Could you check a few things on this model? Use its own coordinates, in mm. Give positions to 0.01 mm unless a question says otherwise; leave off trailing zeros. Loops run counter-clockwise (first coordinate to the right, second up) from the corner with the lowest first, then second, coordinate; pieces in that order, holes last. Notation, with made-up numbers: M 44.5,43.5 L 60.5,43.5 A23 cw 60.5,51.5 Z; hole C 76.25,65 d5. An arc over 180 degrees is marked long. Answer in a Markdown table with one row per item. Add a question column.
1. I'm going to push flat-ended pins straight in: pin 1 Ø1 at (y, z) = (1, -4) entering from -X; pin 2 Ø1.5 at (x, z) = (5.5, -2.5) entering from -Y; pin 3 Ø1 at (y, z) = (2.5, -6.5) entering from +X. Where does each tip first touch, or does it pass through?
2. If we section it at D-D on x = 16: List the corners of the cut face in (y, z) for me, then the cut area to 3 significant figures.
3. I need wall thicknesses on line 1 along X through (y, z) = (1.8, 0); line 2 along X through (y, z) = (1.9, 1.5); line 3 along Z through (x, y) = (-16.5, 1.75). Which ranges of each line are inside material? Lowest first, please. Write a range as from..to.
4. If we section it at B-B on z = 0: List the corners of the cut face in (x, y) for me, then the cut area to 4 significant figures.
5. Thinking about a two-plate mould opening in X: for faces 1 (the cylindrical face through (19.83, 1.52, -8.44)), 2 (the cylindrical face through (19, 2, 0)), 3 (the cylindrical face through (-19.83, 1.52, -8.44)), which applies, released by +X, released by -X, zero draft, split by the parting line, or undercut?
6. If we section it at A-A on y = 1.3: List the corners of the cut face in (x, z) for me, then the cut area to 3 significant figures.
7. If we section it at C-C on x = -18: List the corners of the cut face in (y, z) for me, then the cut area to 3 significant figures.
```python
from build123d import *

# Parameters (mm, degrees)
ESBO_O1_W                = 44.5
ESBO_O1_H                = 22
RESSALTO_EXTRUS_O1_DEPTH = 3
FILETE1_R                = 8.5
ESBO_O2_R                = 2
CORTE_EXTRUS_O1_DEPTH    = 26.001249969


with BuildPart() as part:
    # Esboço1 → Ressalto-extrusão1 (new body)
    with BuildSketch(Plane(origin=(0, 0, 0), x_dir=(1, 0, 0), z_dir=(0, 1, 0))):
        Rectangle(ESBO_O1_W, ESBO_O1_H)
    extrude(amount=RESSALTO_EXTRUS_O1_DEPTH)

    # Filete1
    filete1_edges = [part.edges().sort_by_distance(p)[0] for p in [
        (22.25, 1.5, 11),
        (-22.25, 1.5, 11),
        (-22.25, 1.5, -11),
        (22.25, 1.5, -11),
    ]]
    fillet(filete1_edges, radius=FILETE1_R)

    # Esboço2 → Corte-extrusão1 (cut, through all)
    with BuildSketch(Plane(origin=(0, 3, 0), x_dir=(1, 0, 0), z_dir=(0, 1, 0))):
        with Locations(Location((-17, 0, 0), (0, 0, 270))):
            Circle(ESBO_O2_R)
        with Locations(Location((17, 0, 0), (0, 0, 270))):
            Circle(ESBO_O2_R)
    extrude(amount=-CORTE_EXTRUS_O1_DEPTH, mode=Mode.SUBTRACT)


solid = part.part
```
Results:
| question | item | result |
|---|---|---|
| 1 | pin 1 | x = -22.19 |
| 1 | pin 2 | y = 0 |
| 1 | pin 3 | x = 21.5 |
| 2 | outline | M 0,-10.7 L 3,-10.7 L 3,-1.73 L 0,-1.73 Z; M 0,1.73 L 3,1.73 L 3,10.7 L 0,10.7 Z |
| 2 | area | 53.8 mm2 |
| 3 | line 1 | -22.25..-19, -15..15, 19..22.25 |
| 3 | line 2 | -22.25..-18.32, -15.68..15.68, 18.32..22.25 |
| 3 | line 3 | -10.54..-1.94, 1.94..10.54 |
| 4 | outline | M -22.25,0 L -19,0 L -19,3 L -22.25,3 Z; M -15,0 L 15,0 L 15,3 L -15,3 Z; M 19,0 L 22.25,0 L 22.25,3 L 19,3 Z |
| 4 | area | 109.5 mm2 |
| 5 | face 1 | released by +X |
| 5 | face 2 | undercut |
| 5 | face 3 | released by -X |
| 6 | outline | M -22.25,-2.5 A8.5 ccw -13.75,-11 L 13.75,-11 A8.5 ccw 22.25,-2.5 L 22.25,2.5 A8.5 ccw 13.75,11 L -13.75,11 A8.5 ccw -22.25,2.5 Z; hole C -17,0 d4; hole C 17,0 d4 |
| 6 | area | 892 mm2 |
| 7 | outline | M 0,-9.86 L 3,-9.86 L 3,-1.73 L 0,-1.73 Z; M 0,1.73 L 3,1.73 L 3,9.86 L 0,9.86 Z |
| 7 | area | 48.8 mm2 |
